```python
from build123d import *

# Parameters (mm, degrees)
SKETCH1_W           = 15.875
SKETCH1_H           = 63.5
BOSS_EXTRUDE1_DEPTH = 38.1
CUT_EXTRUDE1_DEPTH  = 16.875
SKETCH3_R           = 6.746875
CUT_EXTRUDE2_DEPTH  = 16.875


with BuildPart() as part:
    # Sketch1 → Boss-Extrude1 (new body)
    with BuildSketch(Plane.XY):
        with Locations((7.9375, 31.75)):
            Rectangle(SKETCH1_W, SKETCH1_H)
    extrude(amount=BOSS_EXTRUDE1_DEPTH)

    # Sketch2 → Cut-Extrude1 (cut, through all)
    with BuildSketch(Plane.ZY):
        with BuildLine():
            ThreePointArc((24.4280023, 38.7985), (20.984165451, 31.75), (24.4280023, 24.7015))
            Line((24.4280023, 24.7015), (38.1, 24.7015))
            Line((38.1, 24.7015), (38.1, 38.7985))
            Line((38.1, 38.7985), (24.4280023, 38.7985))
        make_face()
    extrude(amount=-CUT_EXTRUDE1_DEPTH, mode=Mode.SUBTRACT)

    # Sketch3 → Cut-Extrude2 (cut, through all)
    with BuildSketch(Plane.ZY):
        with Locations((12.7, 51.14925)):
            Circle(SKETCH3_R)
        with Locations((12.7, 12.7)):
            Circle(SKETCH3_R)
    extrude(amount=-CUT_EXTRUDE2_DEPTH, mode=Mode.SUBTRACT)


solid = part.part
```
The model under review builds one solid part; all positions refer to its coordinate system, in mm. A direction names the side the tool comes from. Round coordinates to 2 decimals unless told otherwise and drop trailing zeros. Loops run counter-clockwise (first coordinate to the right, second up) from the corner with the lowest first, then second, coordinate; pieces in that order, holes last. Notation, with made-up numbers: (-7, 35.25) -> (43, 35.25) arc R22 cw to (43, 44.25) -> close; hole circle Ø3 at (45.25, -19). An arc over 180 degrees is marked (long way). Answer as a JSON object with one key per item and string values. Group by question number.
1) We need section C-C on z = 35. Write out the cut boundary in (x, y) (1 decimal), then the cut area to 3 significant figures.
2) For line 1 (Y direction, x = 4.25, z = 12.7); line 2 (Y direction, x = 8, z = 14); line 3 (Y direction, x = 4.25, z = 29), list the stretches that pass through material, from the lowest coordinate up. Write a range as [from, to].
3) For faces 5 (the face through (8, 24.702, 31)), 6 (the face through (8, 51, 38.1)), list the 3-axis set-ups (+Z, -Z, +X, -X, +Y, -Y) from which the entire face can be reached by the end or side of a thin tool; tool diameter is ignored.
4) We need section B-B on y = 12.7. Write out the cut boundary in (x, z) (3 decimals), then the cut area to 3 significant figures.
5) We need section A-A on z = 12.7. Write out the cut boundary in (x, y) (3 decimals), then the cut area to 3 significant figures.
6) We need section D-D on x = 11.5. Give the number of separate pieces and of enclosed holes in the cut face, then the cut area to 3 significant figures.
7) Mouldability with a two-part tool opening along Z and no side actions: class faces 1 (the face through (7.826, 10.116, 18.932)), 2 (the face through (7.826, 56.838, 16.327)), 3 (the face through (8, 0, 19)), 4 (the face through (7.826, 31.864, 20.985)) as released by +Z, released by -Z, zero draft, split by the parting line, or undercut.
Result set:
{
 "1": {"outline": "(0, 0) -> (15.9, 0) -> (15.9, 24.7) -> (0, 24.7) -> close; (0, 38.8) -> (15.9, 38.8) -> (15.9, 63.5) -> (0, 63.5) -> close", "area": "784 mm²"},
 "2": {"line 1": "[0, 5.95], [19.45, 44.4], [57.9, 63.5]", "line 2": "[0, 6.08], [19.32, 44.53], [57.77, 63.5]", "line 3": "[0, 24.7], [38.8, 63.5]"},
 "3": {"face 5": "+Z, +X, -X", "face 6": "+Z, +X, -X, +Y, -Y"},
 "4": {"outline": "(0, 0) -> (15.875, 0) -> (15.875, 5.953) -> (0, 5.953) -> close; (0, 19.447) -> (15.875, 19.447) -> (15.875, 38.1) -> (0, 38.1) -> close", "area": "391 mm²"},
 "5": {"outline": "(0, 0) -> (15.875, 0) -> (15.875, 5.953) -> (0, 5.953) -> close; (0, 19.447) -> (15.875, 19.447) -> (15.875, 44.402) -> (0, 44.402) -> close; (0, 57.896) -> (15.875, 57.896) -> (15.875, 63.5) -> (0, 63.5) -> close", "area": "580 mm²"},
 "6": {"separate pieces": "1", "enclosed holes": "2", "area": "1,910 mm²"},
 "7": {"face 1": "undercut", "face 2": "undercut", "face 3": "zero draft", "face 4": "released by +Z"}
}
